from build123d import *

# Parameters (mm, degrees)
SKETCH1_R           = 11
SKETCH1_R_2         = 9.5
BOSS_EXTRUDE1_DEPTH = 2
EXTRUDE_THIN1_DEPTH = 8
CUT_EXTRUDE1_START  = -6
SKETCH3_R           = 9.5
CUT_EXTRUDE1_DEPTH  = 6


with BuildPart() as part:
    # Sketch1 → Boss-Extrude1 (new body)
    with BuildSketch(Plane(origin=(0, 2, 0), x_dir=(1, 0, 0), z_dir=(0, 1, 0))):
        with Locations(Location((0, 0, 0), (0, 0, 270))):
            Circle(SKETCH1_R)
        with Locations(Location((0, 0, 0), (0, 0, 270))):
            Circle(SKETCH1_R_2, mode=Mode.SUBTRACT)
    extrude(amount=-BOSS_EXTRUDE1_DEPTH)

    # Sketch2 → Extrude-Thin1 (add)
    with BuildSketch(Plane(origin=(0, 2, 0), x_dir=(1, 0, 0), z_dir=(0, 1, 0))):
        Polygon((-23.960036171, -43.5), (10.68097998, 16.5), (8.948929172, 17.5), (-25.692086979, -42.5), align=None)
        Polygon((-10.68097998, 16.5), (23.960036171, -43.5), (25.692086979, -42.5), (-8.948929172, 17.5), align=None)
    extrude(amount=EXTRUDE_THIN1_DEPTH)

    # Sketch3 → Cut-Extrude1 (cut)
    with BuildSketch(Plane.XZ.offset(CUT_EXTRUDE1_START)):
        with Locations(Location((0, 0, 0), (0, 0, 90))):
            Circle(SKETCH3_R)
    extrude(amount=CUT_EXTRUDE1_DEPTH, mode=Mode.SUBTRACT)


solid = part.part
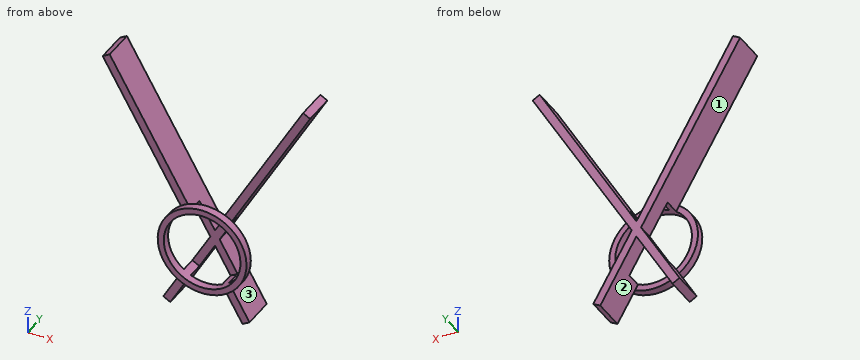
Input: part model. Units: mm. Frame: model coordinates. Face numbers are marked on the shaded views. Coordinates: 2 decimals unless noted, no trailing zeros. Loops run counter-clockwise (first coordinate to the right, second up) from the corner with the lowest first, then second, coordinate; pieces in that order, holes last. Notation, with made-up numbers: (30.25, -7.5) -> (36.25, -7.5) arc R6 ccw to (36.25, -3.5) -> close; hole circle Ø1 at (-8, -21.5). An arc over 180 degrees is marked (long way). Write each question's results on one line, items separated by ' | '. Start each with the question number.
Q1. Section A-A, the plane z = 30. Return the cut outline in (x, y), plus the area to 3 significant figures.
Q2. Section B-B, the plane y = 3.75. Return the cut outline in (x, z), plus the area to 3 significant figures.
Q3. Section D-D, the plane x = -22. Return the cut outline in (y, z).
Q4. Pin query (flat end, axial travel): pin 1 (17 mm diameter, centred on x = -10.5, z = 24, fed in from -Y); pin 2 (1 mm diameter, centred on x = -7.5, y = 7.5, fed in from -Z); pin 3 (4.5 mm diameter, centred on x = -9, z = -3, fed in from +Y). Return the tip coordinate at first contact, or that it passes through.
Q5. Pull-direction query (X, two-part tool) for the marked faces 1, 2 and 3; classes: released by +X, released by -X, zero draft, split by the parting line, or undercut.
Q6. Section C-C, the plane y = 8.5. Return the cut outline in (x, z).
Q7. Ray query, line 1 (Z direction, x = 0, y = 1.35); line 2 (X direction, y = 2.75, z = 26.5); line 3 (X direction, y = 7, z = 25.5). Return the intervals inside material, ascending. Write a range as from..to.
Found:
1) outline: (-18.48, 2) -> (-16.17, 2) -> (-16.17, 10) -> (-18.48, 10) -> close; (16.17, 2) -> (18.48, 2) -> (18.48, 10) -> (16.17, 10) -> close | area: 37.0 mm2
2) outline: (-25.69, 42.5) -> (-5.59, 7.68) arc R9.5 cw to (-3.86, 8.68) -> (-23.96, 43.5) -> close; (-10.68, -16.5) -> (-8.95, -17.5) -> (-3.86, -8.68) arc R9.5 cw to (-5.59, -7.68) -> close; (3.86, -8.68) -> (8.95, -17.5) -> (10.68, -16.5) -> (5.59, -7.68) arc R9.5 cw to start; (3.86, 8.68) arc R9.5 cw to (5.59, 7.68) -> (25.69, 42.5) -> (23.96, 43.5) -> close | area: 201 mm2
3) outline: (2, 36.11) -> (10, 36.11) -> (10, 40.11) -> (2, 40.11) -> close
4) pin 1: y = 2 | pin 2: z = -15.86 | pin 3: y = 2
5) face 1: released by -X | face 2: undercut | face 3: released by +X
6) outline: (-25.69, 42.5) -> (-1.15, 0) -> (-10.68, -16.5) -> (-8.95, -17.5) -> (0, -2) -> (8.95, -17.5) -> (10.68, -16.5) -> (1.15, 0) -> (25.69, 42.5) -> (23.96, 43.5) -> (0, 2) -> (-23.96, 43.5) -> close
7) line 1: -11..-9.5, 9.5..11 | line 2: -16.45..-14.15, 14.15..16.45 | line 3: -15.88..-13.57, 13.57..15.88
